Model file for the job. Use its own axes, mm. Round coordinates to 2 decimals unless told otherwise and drop trailing zeros. Loops run counter-clockwise (first coordinate to the right, second up) from the corner with the lowest first, then second, coordinate; pieces in that order, holes last.
from build123d import *

# Parameters (mm, degrees)
SKETCH1_W           = 190.5
SKETCH1_H           = 304.8
BOSS_EXTRUDE1_DEPTH = 2.778125
SKETCH2_W           = 190.5
SKETCH2_H           = 17.78
CUT_EXTRUDE1_DEPTH  = 3.778125
SKETCH3_W           = 17.78
SKETCH3_H           = 269.24
CUT_EXTRUDE2_DEPTH  = 3.778125
CUT_EXTRUDE3_DEPTH  = 3.778125
SKETCH5_W           = 10.16
SKETCH5_H           = 10.16
CUT_EXTRUDE4_DEPTH  = 3.778125
FILLET1_R           = 2.54


with BuildPart() as part:
    # Sketch1 → Boss-Extrude1 (new body)
    with BuildSketch(Plane(origin=(0, 0, 0), x_dir=(1, 0, 0), z_dir=(0, 1, 0))):
        with Locations((95.25, 152.4)):
            Rectangle(SKETCH1_W, SKETCH1_H)
    extrude(amount=BOSS_EXTRUDE1_DEPTH)

    # Sketch2 → Cut-Extrude1 (cut, through all)
    with BuildSketch(Plane(origin=(0, 2.778125, 0), x_dir=(1, 0, 0), z_dir=(0, 1, 0))):
        with Locations((95.25, 8.89)):
            Rectangle(SKETCH2_W, SKETCH2_H)
        with Locations((95.25, 295.91)):
            Rectangle(SKETCH2_W, SKETCH2_H)
    extrude(amount=-CUT_EXTRUDE1_DEPTH, mode=Mode.SUBTRACT)

    # Sketch3 → Cut-Extrude2 (cut, through all)
    with BuildSketch(Plane(origin=(0, 2.778125, 0), x_dir=(1, 0, 0), z_dir=(0, 1, 0))):
        with Locations((8.89, 152.4)):
            Rectangle(SKETCH3_W, SKETCH3_H)
    extrude(amount=-CUT_EXTRUDE2_DEPTH, mode=Mode.SUBTRACT)

    # Sketch4 → Cut-Extrude3 (cut, through all)
    with BuildSketch(Plane(origin=(0, 2.778125, 0), x_dir=(1, 0, 0), z_dir=(0, 1, 0))):
        Polygon((22.86, 252.73), (44.45, 274.32), (44.45, 287.02), (17.78, 287.02), (17.78, 252.73), align=None)
        Polygon((22.86, 52.07), (44.45, 30.48), (44.45, 17.78), (17.78, 17.78), (17.78, 52.07), align=None)
    extrude(amount=-CUT_EXTRUDE3_DEPTH, mode=Mode.SUBTRACT)

    # Sketch5 → Cut-Extrude4 (cut, through all)
    with BuildSketch(Plane(origin=(0, 2.778125, 0), x_dir=(1, 0, 0), z_dir=(0, 1, 0))):
        with Locations((185.42, 281.94)):
            Rectangle(SKETCH5_W, SKETCH5_H)
        with Locations((185.42, 22.86)):
            Rectangle(SKETCH5_W, SKETCH5_H)
    extrude(amount=-CUT_EXTRUDE4_DEPTH, mode=Mode.SUBTRACT)

    # Fillet1
    fillet1_edges = [part.edges().sort_by_distance(p)[0] for p in [
        (190.5, 1.3890625, -27.94),
        (180.34, 1.3890625, -17.78),
        (180.34, 1.3890625, -27.94),
        (44.45, 1.3890625, -287.02),
        (44.45, 1.3890625, -274.32),
        (22.86, 1.3890625, -252.73),
        (17.78, 1.3890625, -252.73),
        (17.78, 1.3890625, -52.07),
        (22.86, 1.3890625, -52.07),
        (44.45, 1.3890625, -30.48),
        (44.45, 1.3890625, -17.78),
        (190.5, 1.3890625, -276.86),
        (180.34, 1.3890625, -276.86),
        (180.34, 1.3890625, -287.02),
    ]]
    fillet(fillet1_edges, radius=FILLET1_R)


solid = part.part
Q1. Slice it at A-A on y = 1. Give the cut face in (x, z).
Q2. Flat gauge pins, fed straight in: P1, Ø0.8, axis at y = 1.5, z = -22, coming from the +X side; P2, Ø1.2, axis at x = 21, y = 1.5, coming from the -Z side; P3, Ø1.4, axis at y = 1, z = -26.5, coming from the -X side. Where does each tip first touch, or does it go through?
Q3. Probe line 1 (Z direction, x = 182.5, y = 1); line 2 (Z direction, x = 30, y = 1.3); line 3 (X direction, y = 0.3, z = -40). List the from-to ranges inside material, lowest first.
Reply:
1. outline: (17.78, -250.19) arc R2.54 ccw to (20.32, -252.73) - (21.81, -252.73) arc R2.54 cw to (23.6, -253.47) - (43.71, -273.58) arc R2.54 cw to (44.45, -275.37) - (44.45, -284.48) arc R2.54 ccw to (46.99, -287.02) - (177.8, -287.02) arc R2.54 ccw to (180.34, -284.48) - (180.34, -279.4) arc R2.54 cw to (182.88, -276.86) - (187.96, -276.86) arc R2.54 ccw to (190.5, -274.32) - (190.5, -30.48) arc R2.54 ccw to (187.96, -27.94) - (182.88, -27.94) arc R2.54 cw to (180.34, -25.4) - (180.34, -20.32) arc R2.54 ccw to (177.8, -17.78) - (46.99, -17.78) arc R2.54 ccw to (44.45, -20.32) - (44.45, -29.43) arc R2.54 cw to (43.71, -31.22) - (23.6, -51.33) arc R2.54 cw to (21.81, -52.07) - (20.32, -52.07) arc R2.54 ccw to (17.78, -54.61) - close
2. P1: stops at x = 180.34
2. P2: stops at z = -252.73
2. P3: stops at x = 44.45
3. line 1: z = -276.89 to -27.91
3. line 2: z = -259.87 to -44.93
3. line 3: x = 34.93 to 190.5
